Design review of the part built by this model. Coordinates are the model's own, in mm. Give positions to 0.01 mm unless a question says otherwise; leave off trailing zeros. Loops run counter-clockwise (first coordinate to the right, second up) from the corner with the lowest first, then second, coordinate; pieces in that order, holes last. Notation, with made-up numbers: M 31,-40 L 82,-40 A31 ccw 82,-5 Z; hole C 77.25,-21 d4. An arc over 180 degrees is marked long. Answer as CSV lines item,"result".
Autodesk Inventor part; units mm, degrees
ref_plane "Work Plane1" through (-60, 0, 3) normal (0, 1, 0) x (1, 0, 0)
ref_plane "YZ Plane" through (0, 0, 0) normal (1, 0, 0) x (0, 1, 0)
ref_plane "XZ Plane" through (0, 0, 0) normal (0, 1, 0) x (-1, 0, 0)
sketch "Sketch1" plane through (0, 0, 0) normal (0, 0, 1) x (1, 0, 0)
  line L0 (-60, 7.5) -> (60, 7.5)
  line L1 (60, 7.5) -> (60, -7.5)
  line L2 (60, -7.5) -> (-60, -7.5)
  line L3 (-60, -7.5) -> (-60, 7.5)
  line L4 (-60, 7.5) -> (60, -7.5) construction
  line L5 (60, 7.5) -> (-60, -7.5) construction
  circle A0 centre (-52.5, 0) radius 2.5
  circle A1 centre (52.5, 0) radius 2.5
  point P0 (0, 0)
  point P1 (-60, 0)
  point P2 (60, 0)
  dimension "d0" = 120
  dimension "d1" = 15
  dimension "d2" = 5
  dimension "d3" = 7.5
  dimension "d4" = 7.5
extrude "Extrusion1" add sketch "Sketch1" along normal blind 3
sketch "Sketch2" plane through (0, 0, 3) normal (0, 0, 1) x (1, 0, 0)
  line L0 (-40, 0) -> (40, 0) construction
  point P0 (0, 0)
  point P1 (0, 0)
  dimension "d7" = 80
hole "Hole1" at (-40, 0, 3) at (40, 0, 3) direction (0, 0, -1) diameter 3.3 depth 36.25 countersink diameter 6.5 countersink angle 90
sketch "Sketch3" plane through (0, 0, 3) normal (0, 0, 1) x (1, 0, 0)
  line L0 (-30, 7.5) -> (30, 7.5)
  line L1 (30, 7.5) -> (30, 4)
  line L2 (30, 4) -> (-30, 4)
  line L3 (-30, 4) -> (-30, 7.5)
  circle A0 centre (-40, 0) radius 1.65
  circle A1 centre (40, 0) radius 1.65
  line L4 (60, 7.5) -> (-60, 7.5)
  point P0 (0, 0)
  dimension "d16" = 10
  dimension "d17" = 10
  dimension "d18" = 4
extrude "Extrusion2" cut sketch "Sketch3" against normal blind 3 contours L0 L1 L2 L3
ref_plane "Work Plane1" through (-60, 0, 3) normal (0, 1, 0) x (1, 0, 0)
mirror "Mirror1" about plane through (-60, 0, 3) normal (0, 1, 0) of "Extrusion2"
fillet "Fillet1" radius 2 12 edges at (-60, 7.5, 1.5) (-60, -7.5, 1.5) (60, 7.5, 1.5) (60, -7.5, 1.5) (-30, 7.5, 1.5) (-30, 4, 1.5) (-30, -4, 1.5) (-30, -7.5, 1.5) (30, 7.5, 1.5) (30, 4, 1.5) (30, -7.5, 1.5) (30, -4, 1.5)
equation "\"d4\" = d3"
equation "\"d17\" = d16"
properties part number "Power Supply Wall Mount v2"
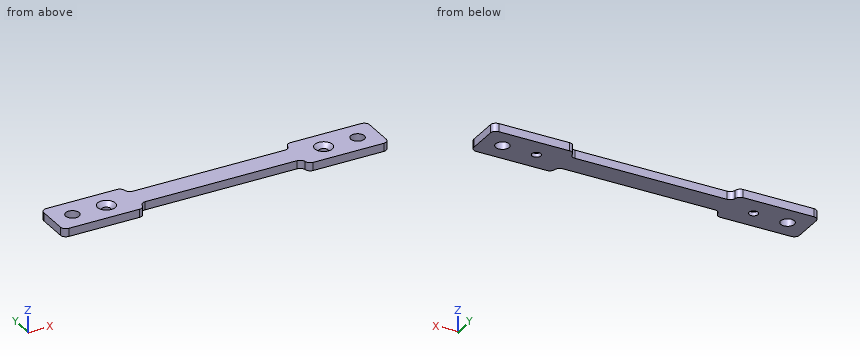
1. For P1, Ø6.5, axis at x = -52.5, y = 0, coming from the -Z side; P2, Ø3, axis at x = 40, y = 0, coming from the -Z side, all flat-tipped, find the tip position at first contact; note any pin that passes through.
Answer block:
P1,"z = 0"
P2,"through"
2. We need section A-A, the plane y = 0. Write out the cut boundary in (x, z).
Answer block:
outline,"M -60,0 L -55,0 L -55,3 L -60,3 Z; M -50,0 L -41.65,0 L -41.65,1.4 L -43.25,3 L -50,3 Z; M -38.35,0 L 38.35,0 L 38.35,1.4 L 36.75,3 L -36.75,3 L -38.35,1.4 Z; M 41.65,0 L 50,0 L 50,3 L 43.25,3 L 41.65,1.4 Z; M 55,0 L 60,0 L 60,3 L 55,3 Z"
3. We need section B-B, the plane x = 52.5. Write out the cut boundary in (y, z).
Answer block:
outline,"M -7.5,0 L -2.5,0 L -2.5,3 L -7.5,3 Z; M 2.5,0 L 7.5,0 L 7.5,3 L 2.5,3 Z"
4. We need section D-D, the plane z = 2.4. Count the separate pieces of the cut face and the enclosed holes in it, plus the area to 3 significant figures.
Answer block:
separate pieces,"1"
enclosed holes,"4"
area,"1,290 mm²"
5. We need section C-C, the plane x = -40. Write out the cut boundary in (y, z), plus the area to 3 significant figures.
Answer block:
outline,"M -7.5,0 L -1.65,0 L -1.65,1.4 L -3.25,3 L -7.5,3 Z; M 1.65,0 L 7.5,0 L 7.5,3 L 3.25,3 L 1.65,1.4 Z"
area,"32.5 mm²"
6. To check wall thickness, follow L1, parallel to Y at x = -52.5, z = 1.25; L2, parallel to X at y = -5.75, z = 0.2; L3, parallel to X at y = 1.75, z = 1.05. State the ranges of each line that lie inside material, in increasing order. Write a range as [from, to].
Answer block:
L1,"[-7.5, -2.5], [2.5, 7.5]"
L2,"[-59.98, -29.98], [30.02, 59.98]"
L3,"[-60, -54.29], [-50.71, 50.71], [54.29, 60]"
